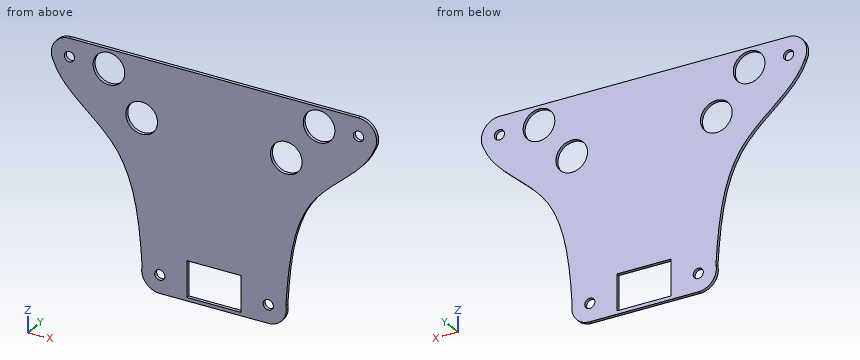
from build123d import *

# Parameters (mm, degrees)
F0_R     = 7.1501
F0_R_2   = 22.2504
F1_DEPTH = 4.7498


with BuildPart() as f1:
    # F0 (on Front) → F1 (new body)
    with BuildSketch(Plane.XZ):
        with BuildLine():
            ThreePointArc((-225.6573369788, 94.4161567678), (-197.0867504248, 81.6298943923), (-177.8, 106.2832548048))
            ThreePointArc((-177.8, 106.2832548048), (-185.2394877579, 124.2437670469), (-203.2, 131.6832548048))
            ThreePointArc((-203.2, 131.6832548048), (-224.9552785565, 119.3930929018), (-225.6573369788, 94.4161567678))
        make_face()
        with Locations((-203.2, 106.2832548048)):
            Circle(F0_R, mode=Mode.SUBTRACT)
        with BuildLine():
            ThreePointArc((-203.2, 131.6832548048), (-185.2394877579, 124.2437670469), (-177.8, 106.2832548048))
            ThreePointArc((-177.8, 106.2832548048), (-197.0867504248, 81.6298943923), (-225.6573369788, 94.4161567678))
            add(Edge.make_bspline(
                [(-225.6573369788, 94.4161567678), (-210.8833649868, 55.9874046479), (-115.4710726931, 10.7964254469), (-104.8309285082, -94.2151341667), (-101.0213270695, -155.0258526432)],
                knots=[0, 0, 0, 0, 0.4720003547, 1, 1, 1, 1], degree=3))
            ThreePointArc((-101.0213270695, -155.0258526432), (-73.4890691235, -135.1618277773), (-50.8, -160.4167451952))
            ThreePointArc((-50.8, -160.4167451952), (-58.2394877579, -178.3772574373), (-76.2, -185.8167451952))
            Line((-76.2, -185.8167451952), (76.2, -185.8167451952))
            ThreePointArc((76.2, -185.8167451952), (56.4251590294, -144.4757394368), (101.0213270695, -155.0258526432))
            add(Edge.make_bspline(
                [(225.6573369788, 94.4161567678), (210.8833649868, 55.9874046479), (115.4710726931, 10.7964254469), (104.8309285082, -94.2151341667), (101.0213270695, -155.0258526432)],
                knots=[0, 0, 0, 0, 0.4720003547, 1, 1, 1, 1], degree=3))
            ThreePointArc((225.6573369788, 94.4161567678), (181.4447214435, 93.1734167078), (203.2, 131.6832548048))
            Line((203.2, 131.6832548048), (-203.2, 131.6832548048))
        make_face()
        Polygon((-38.1, -130.2669451952), (0, -130.2669451952), (38.1, -130.2669451952), (38.1, -181.0669451952), (0, -181.0669451952), (-38.1, -181.0669451952), align=None, mode=Mode.SUBTRACT)
        with Locations((-101.6, 49.1332548048)):
            Circle(F0_R_2, mode=Mode.SUBTRACT)
        with Locations((-147.6502, 104.6830548048)):
            Circle(F0_R_2, mode=Mode.SUBTRACT)
        with Locations((101.6, 49.1332548048)):
            Circle(F0_R_2, mode=Mode.SUBTRACT)
        with Locations((147.6502, 104.6830548048)):
            Circle(F0_R_2, mode=Mode.SUBTRACT)
        with BuildLine():
            ThreePointArc((228.6, 106.2832548048), (221.1605122421, 124.2437670469), (203.2, 131.6832548048))
            ThreePointArc((203.2, 131.6832548048), (181.4447214435, 93.1734167078), (225.6573369788, 94.4161567678))
            ThreePointArc((225.6573369788, 94.4161567678), (227.8533604125, 100.1700052296), (228.6, 106.2832548048))
        make_face()
        with Locations((203.2, 106.2832548048)):
            Circle(F0_R, mode=Mode.SUBTRACT)
        with BuildLine():
            ThreePointArc((-50.8, -160.4167451952), (-73.4890691235, -135.1618277773), (-101.0213270695, -155.0258526432))
            ThreePointArc((-101.0213270695, -155.0258526432), (-95.9748409706, -176.3577509536), (-76.2, -185.8167451952))
            ThreePointArc((-76.2, -185.8167451952), (-58.2394877579, -178.3772574373), (-50.8, -160.4167451952))
        make_face()
        with Locations((-76.2, -160.4167451952)):
            Circle(F0_R, mode=Mode.SUBTRACT)
        with BuildLine():
            ThreePointArc((101.6, -160.4167451952), (101.4549174179, -157.7058143187), (101.0213270695, -155.0258526432))
            ThreePointArc((101.0213270695, -155.0258526432), (56.4251590294, -144.4757394368), (76.2, -185.8167451952))
            ThreePointArc((76.2, -185.8167451952), (94.1605122421, -178.3772574373), (101.6, -160.4167451952))
        make_face()
        with Locations((76.2, -160.4167451952)):
            Circle(F0_R, mode=Mode.SUBTRACT)
    extrude(amount=F1_DEPTH)


solid = f1.part
Source: CAD feature listing. Evaluate the final solid. Frame: model axes, mm. Round coordinates to 2 decimals unless told otherwise and drop trailing zeros. Write each loop counter-clockwise with the first axis right and the second up, starting at its lowest first coordinate (ties: lowest second). Pieces come first, ordered by that corner, then holes. Notation, with made-up numbers: (66, 2.5) - (89, 2.5) arc R24 ccw to (89, 37.5) - close; hole circle Ø10 at (52.25, 5). An arc over 180 degrees is marked (long way). Use CSV: the item, a comma, the result in double quotes. Start each with the question number.
(1) First-contact query: pin 1 Ø2.5 at (y, z) = (-2.5, -145.5) entering from -X; pin 2 Ø2 at (y, z) = (-2, -97) entering from +X. Flat tips, straight axial feed; report the tip coordinate or a pass-through.
(2) Cut plane B-B, the plane y = -3.2. Give the number of separate pieces and of enclosed holes in the cut face, and give its area (3 significant figures).
(3) Cut plane A-A, the plane x = 90. Return loops of the section in (y, z), and give its area (3 significant figures).
(4) Material intervals for probe 1 along Z at (x, y) = (-76.2, -2.2); probe 2 along X at (y, z) = (-2.65, 59); probe 3 along Z at (x, y) = (6.5, -3.35), sorted ascending. Write a range as [from, to].
Geometry says:
1,pin 1,"x = -101.72"
1,pin 2,"x = 106.3"
2,separate pieces,"1"
2,enclosed holes,"9"
2,area,"82,100 mm²"
3,outline,"(-4.75, -181.74) - (0, -181.74) - (0, 30.15) - (-4.75, 30.15) - close; (-4.75, 68.12) - (0, 68.12) - (0, 131.68) - (-4.75, 131.68) - close"
3,area,"1,310 mm²"
4,probe 1,"[-185.82, -167.57], [-153.27, 131.68]"
4,probe 2,"[-201.09, -121.54], [-81.66, 81.66], [121.54, 201.09]"
4,probe 3,"[-185.82, -181.07], [-130.27, 131.68]"
